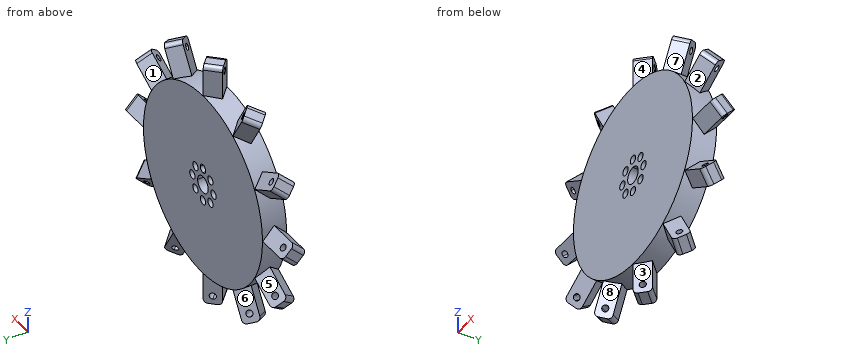
```python
from build123d import *

# Parameters (mm, degrees)
F2_W            = 4
F2_H            = 60
F3_DEPTH        = 4
F3_COPIES_COUNT = 12
F4_R            = 45
F5_DEPTH        = 5.75
F7_DEPTH        = 25
F7_COPIES_COUNT = 12
F8_R            = 2
F9_R            = 2
F10_DEPTH       = 25


# Not quite as in the source:
# - a pattern or mirror of a feature is missing from the dataset's text; its kind, count and spacing are read off the source's solid


with BuildPart() as f3:
    # F2 (on face) → F3 (new body, symmetric)
    with BuildSketch(Plane(origin=(0, 0, 0), x_dir=(-0.7071067812, 0.7071067812, 0), z_dir=(0.7071067812, 0.7071067812, 0))):
        with Locations((-2, 30)):
            Rectangle(F2_W, F2_H)
        with Locations((2, 30)):
            Rectangle(F2_W, F2_H)
    extrude(amount=F3_DEPTH, both=True)

    # F3_copies: F3 ×12 about axis
    f3_copies_axis = Axis((0, 0, 0), (0, 1, 0))


with BuildPart() as f3_1:
    add(f3.part)
    for i in range(1, F3_COPIES_COUNT):
        add(f3.part.rotate(f3_copies_axis, i * 360 / F3_COPIES_COUNT))

    # F4 (on Front) → F5 (join, symmetric)
    with BuildSketch(Plane.XZ):
        Circle(F4_R)
    extrude(amount=F5_DEPTH, both=True)

    # F6 (on face) → F7 (cut)
    with BuildSketch(Plane(origin=(-2.8284271247, -2.8284271247, 0), x_dir=(0.7071067812, -0.7071067812, 0), z_dir=(-0.7071067812, -0.7071067812, 0))):
        with BuildLine():
            ThreePointArc((1.5, 56), (1.0606601718, 57.0606601718), (0, 57.5))
            ThreePointArc((0, 57.5), (-1.0606601718, 54.9393398282), (1.5, 56))
        make_face()
    f7 = extrude(amount=-F7_DEPTH, mode=Mode.SUBTRACT)

    # F7_copies: F7 ×12 about axis
    f7_copies_axis = Axis((0, 0, 0), (0, 1, 0))
    for i in range(1, F7_COPIES_COUNT):
        add(f7.rotate(f7_copies_axis, i * 360 / F7_COPIES_COUNT), mode=Mode.SUBTRACT)

    # F8
    f8_edges = [f3_1.edges().sort_by_distance(p)[0] for p in [
        (2.828427, -2.828427, 60),
        (-2.828427, 2.828427, 60),
        (60, 2.828427, 2.828427),
        (60, -2.828427, -2.828427),
        (53.375738, -2.828427, 27.55051),
        (50.547311, 2.828427, 32.44949),
        (32.44949, -2.828427, 50.547311),
        (27.55051, 2.828427, 53.375738),
        (-32.44949, 2.828427, 50.547311),
        (-27.55051, -2.828427, 53.375738),
        (-53.375738, 2.828427, 27.55051),
        (-50.547311, -2.828427, 32.44949),
        (-60, 2.828427, -2.828427),
        (-60, -2.828427, 2.828427),
        (-50.547311, 2.828427, -32.44949),
        (-53.375738, -2.828427, -27.55051),
        (-27.55051, 2.828427, -53.375738),
        (-32.44949, -2.828427, -50.547311),
        (27.55051, -2.828427, -53.375738),
        (32.44949, 2.828427, -50.547311),
        (50.547311, -2.828427, -32.44949),
        (53.375738, 2.828427, -27.55051),
        (2.828427, 2.828427, -60),
        (-2.828427, -2.828427, -60),
    ]]
    fillet(f8_edges, radius=F8_R)

    # F9 (on face) → F10 (cut)
    with BuildSketch(Plane.XZ.offset(5.75)):
        with BuildLine():
            ThreePointArc((0, 4), (-2.8284271247, -2.8284271247), (4, 0))
            ThreePointArc((4, 0), (2.8284271247, 2.8284271247), (0, 4))
        make_face()
        with BuildLine():
            ThreePointArc((2, 8), (-1.4142135624, 9.4142135624), (0, 6))
            ThreePointArc((0, 6), (1.4142135624, 6.5857864376), (2, 8))
        make_face()
        with Locations((-5.6568542495, 5.6568542495)):
            Circle(F9_R)
        with Locations((-8, 0)):
            Circle(F9_R)
        with Locations((-5.6568542495, -5.6568542495)):
            Circle(F9_R)
        with Locations((0, -8)):
            Circle(F9_R)
        with Locations((5.6568542495, -5.6568542495)):
            Circle(F9_R)
        with Locations((8, 0)):
            Circle(F9_R)
        with Locations((5.6568542495, 5.6568542495)):
            Circle(F9_R)
    extrude(amount=-F10_DEPTH, mode=Mode.SUBTRACT)


solid = f3_1.part
```
For this review, take the finished solid that the model builds, in its own axes (mm). Face numbers are marked on the shaded views. A direction names the side the tool comes from. Round coordinates to 2 decimals unless told otherwise and drop trailing zeros. Write each loop counter-clockwise with the first axis right and the second up, starting at its lowest first coordinate (ties: lowest second). Pieces come first, ordered by that corner, then holes. Notation, with made-up numbers: (25, -9.5) -> (42, -9.5) arc R22 ccw to (42, -1.5) -> close; hole circle Ø7 at (-38, 35.25). An arc over 180 degrees is marked (long way). One line per question, with ' | ' between items. Start each with the question number.
(1) Mouldability with a two-part tool opening along X and no side actions: class the marked faces 6, 7 and 8 as released by +X, released by -X, zero draft, split by the parting line, or undercut.
(2) Tool access review of the marked faces 1, 2, 3, 4 and 5: name each direction out of +Z, -Z, +X, -X, +Y, -Y from which nothing blocks a thin tool from reaching the whole face with its end or side.
(3) Add section A-A, the plane z = 43. Write out the cut boundary in (x, y).
(4) Add section C-C, the plane x = 14. Write out the cut boundary in (y, z), plus the area to 3 significant figures.
(5) For line 1 along Z through (x, y) = (0, -2.75); line 2 along X through (y, z) = (-2.75, -29); line 3 along Z through (x, y) = (41, 3.25), list the stretches that pass through material, from the lowest coordinate up. Write a range as from..to.
(6) Insertion check: P1, Ø1.5, axis at x = -28, z = 47.5, coming from the +Y side; P2, Ø3, axis at x = -2, y = 1, coming from the +Z side; P3, Ø2, axis at y = 0.5, z = -25.5, coming from the -X side; P4, Ø1, axis at x = -12.5, y = 2.5, coming from the -Z side. Each pin has a flat end and moves straight along its axis. Give the tip position at first contact, or say it passes through.
(7) Add section B-B, the plane x = -20.5. Write out the cut boundary in (y, z), plus the area to 3 significant figures.
Answer list:
1) face 6: released by -X | face 7: released by +X | face 8: undercut
2) face 1: +Z, +Y | face 2: +X, -Y | face 3: -Z, -Y | face 4: +Z, -Y | face 5: -X, +Y
3) outline: (-31.36, 0) -> (-24.83, -5.66) -> (-18.29, 0) -> (-24.83, 5.66) -> close; (-13.27, -5.75) -> (13.27, -5.75) -> (13.27, 5.75) -> (-13.27, 5.75) -> close; (18.29, 0) -> (24.83, -5.66) -> (31.36, 0) -> (24.83, 5.66) -> close
4) outline: (-5.75, -42.77) -> (5.75, -42.77) -> (5.75, 42.77) -> (-5.75, 42.77) -> close | area: 984 mm²
5) line 1: -60..-10, -6..-4, 4..6, 10..60 | line 2: -52.39..-48.62, -46.31..-44.42, -34.41..34.41, 44.42..52.54 | line 3: -26.45..-20.89, -18.55..18.55, 20.89..26.45
6) P1: y = 5.66 | P2: z = 60 | P3: x = -54.22 | P4: z = -43.37
7) outline: (-5.75, -40.06) -> (-3.38, -40.06) -> (0, -46.82) -> (3.38, -40.06) -> (5.75, -40.06) -> (5.75, 40.06) -> (3.38, 40.06) -> (0, 46.82) -> (-3.38, 40.06) -> (-5.75, 40.06) -> close | area: 967 mm²
